Part model, mm, in its own coordinate system. Face numbers are marked on the shaded views. A direction names the side the tool comes from. Round coordinates to 2 decimals unless told otherwise and drop trailing zeros. Order: outer loops, then holes, each group sorted by start corner. A loop starts at its lowest first (then second) coordinate and runs counter-clockwise, first axis right, second up. Notation, with made-up numbers: (-25, 75) -> (33, 75) arc R9 cw to (33, 87) -> close; hole circle Ø7 at (-11, 72.25). An arc over 180 degrees is marked (long way). Use CSV: the item, a comma, the result in double quotes.
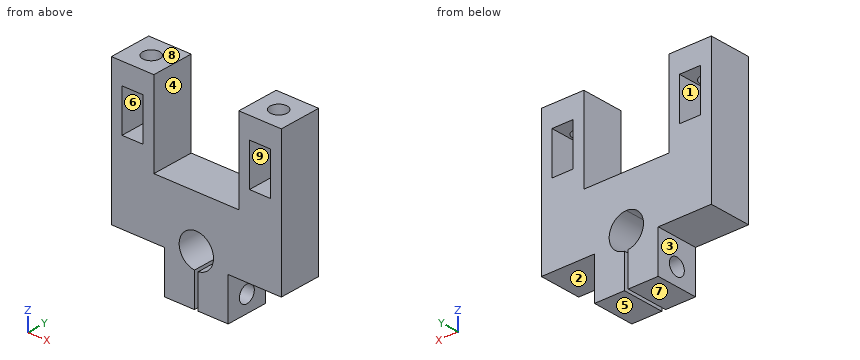
```python
from build123d import *

# Parameters (mm, degrees)
BOSS_EXTRUDE1_DEPTH = 10
SKETCH2_R           = 2
CUT_EXTRUDE1_DEPTH  = 15
SKETCH3_R           = 2
CUT_EXTRUDE2_DEPTH  = 11
SKETCH4_W           = 40
SKETCH4_H           = 24
BOSS_EXTRUDE2_DEPTH = 10
SKETCH5_R           = 4.04
CUT_EXTRUDE3_DEPTH  = 41.693979899
SKETCH6_W           = 0.9
SKETCH6_H           = 12
CUT_EXTRUDE4_DEPTH  = 41.693979899
SKETCH8_R           = 2
CUT_EXTRUDE5_DEPTH  = 40
SKETCH9_W           = 12.5
SKETCH9_H           = 10
CUT_EXTRUDE6_DEPTH  = 40
SKETCH10_W          = 5
SKETCH10_H          = 10
CUT_EXTRUDE7_DEPTH  = 10


with BuildPart() as part:
    # Sketch1 → Boss-Extrude1 (new body)
    with BuildSketch(Plane(origin=(0, 0, 0), x_dir=(1, 0, 0), z_dir=(0, 1, 0))):
        Polygon((-20, -10), (-20, 20), (20, 20), (20, -10), (10, -10), (10, 10), (-10, 10), (-10, -10), align=None)
    extrude(amount=BOSS_EXTRUDE1_DEPTH)

    # Sketch2 → Cut-Extrude1 (cut)
    with BuildSketch(Plane.XY.offset(10)):
        with Locations((-15, 5)):
            Circle(SKETCH2_R)
        with Locations((15, 5)):
            Circle(SKETCH2_R)
    extrude(amount=-CUT_EXTRUDE1_DEPTH, mode=Mode.SUBTRACT)

    # Sketch3 → Cut-Extrude2 (cut)
    with BuildSketch(Plane.XY.offset(-10)):
        with Locations((0, 5)):
            Circle(SKETCH3_R)
    extrude(amount=-CUT_EXTRUDE2_DEPTH, mode=Mode.SUBTRACT)

    # Sketch4 → Boss-Extrude2 (add, through all)
    with BuildSketch(Plane(origin=(0, 10, 0), x_dir=(1, 0, 0), z_dir=(0, 1, 0))):
        with Locations((0, 22)):
            Rectangle(SKETCH4_W, SKETCH4_H)
    extrude(amount=-BOSS_EXTRUDE2_DEPTH)

    # Sketch5 → Cut-Extrude3 (cut, through all)
    with BuildSketch(Plane(origin=(0, 10, 0), x_dir=(1, 0, 0), z_dir=(0, 1, 0))):
        with Locations(Location((0, 22, 0), (0, 0, 270))):
            Circle(SKETCH5_R)
    extrude(amount=-CUT_EXTRUDE3_DEPTH, mode=Mode.SUBTRACT)

    # Sketch6 → Cut-Extrude4 (cut, through all)
    with BuildSketch(Plane(origin=(0, 10, 0), x_dir=(1, 0, 0), z_dir=(0, 1, 0))):
        with Locations((0, 28)):
            Rectangle(SKETCH6_W, SKETCH6_H)
    extrude(amount=-CUT_EXTRUDE4_DEPTH, mode=Mode.SUBTRACT)

    # Sketch8 → Cut-Extrude5 (cut)
    with BuildSketch(Plane.ZY.offset(20)):
        with Locations((-30, 5)):
            Circle(SKETCH8_R)
    extrude(amount=-CUT_EXTRUDE5_DEPTH, mode=Mode.SUBTRACT)

    # Sketch9 → Cut-Extrude6 (cut)
    with BuildSketch(Plane(origin=(0, 10, 0), x_dir=(1, 0, 0), z_dir=(0, 1, 0))):
        with Locations((13.75, 29)):
            Rectangle(SKETCH9_W, SKETCH9_H)
        with Locations((-13.75, 29)):
            Rectangle(SKETCH9_W, SKETCH9_H)
    extrude(amount=-CUT_EXTRUDE6_DEPTH, mode=Mode.SUBTRACT)

    # Sketch10 → Cut-Extrude7 (cut)
    with BuildSketch(Plane(origin=(0, 10, 0), x_dir=(1, 0, 0), z_dir=(0, 1, 0))):
        with Locations((-15, 0)):
            Rectangle(SKETCH10_W, SKETCH10_H)
        with Locations((15, 0)):
            Rectangle(SKETCH10_W, SKETCH10_H)
    extrude(amount=-CUT_EXTRUDE7_DEPTH, mode=Mode.SUBTRACT)


solid = part.part
```
(1) Cut at B-B, the plane y = 7.75. Give the cut face in (x, z), then the cut area to 3 significant figures.
Reply:
outline,"(-20, -24) -> (-7.5, -24) -> (-7.5, -34) -> (-0.45, -34) -> (-0.45, -26.01) arc R4.04 cw (long way) to (0.45, -26.01) -> (0.45, -34) -> (7.5, -34) -> (7.5, -24) -> (20, -24) -> (20, 10) -> (10, 10) -> (10, -10) -> (-10, -10) -> (-10, 10) -> (-20, 10) -> close; hole (-17.5, -5) -> (-12.5, -5) -> (-12.5, 5) -> (-17.5, 5) -> close; hole (12.5, -5) -> (17.5, -5) -> (17.5, 5) -> (12.5, 5) -> close"
area,"952 mm2"
(2) Cut at A-A, the plane z = -9. Give the cut face in (x, y).
Reply:
outline,"(-20, 0) -> (-10, 0) -> (-10, 10) -> (-20, 10) -> close; (10, 0) -> (20, 0) -> (20, 10) -> (10, 10) -> close"
(3) Cut at D-D, the plane z = -30. Give the cut face in (x, y), then the cut area to 3 significant figures.
Reply:
outline,"(-7.5, 0) -> (-0.45, 0) -> (-0.45, 3) -> (-7.5, 3) -> close; (-7.5, 7) -> (-0.45, 7) -> (-0.45, 10) -> (-7.5, 10) -> close; (0.45, 0) -> (7.5, 0) -> (7.5, 3) -> (0.45, 3) -> close; (0.45, 7) -> (7.5, 7) -> (7.5, 10) -> (0.45, 10) -> close"
area,"84.6 mm2"
(4) Drop flat-ended pins along their axis: P1, Ø1, axis at x = -1.5, z = -14.5, coming from the -Y side; P2, Ø3, axis at x = -12.5, y = 4.5, coming from the -Z side. Give the stop position or say it passes through.
Reply:
P1,"y = 0"
P2,"z = -24"
(5) Cut at C-C, the plane x = 15. Give the cut face in (y, z).
Reply:
outline,"(0, -24) -> (10, -24) -> (10, -5) -> (0, -5) -> close; (0, 5) -> (3, 5) -> (3, 10) -> (0, 10) -> close; (7, 5) -> (10, 5) -> (10, 10) -> (7, 10) -> close"
(6) Which spindle directions (+Z, -Z, +X, -X, +Y, -Y) get a long thin tool onto all of the face, cutting with end or side? Do the marked faces 1, 2, 3, 4 and 5. Say none if no direction does.
Reply:
face 1,"+Y, -Y"
face 2,"-Z, +X, +Y, -Y"
face 3,"-Z, -X, +Y, -Y"
face 4,"+Z, +Y, -Y"
face 5,"-Z, +X, -X, +Y, -Y"
(7) Probe probe 1 along X at (y, z) = (3.75, 0.5); probe 2 along X at (y, z) = (9.25, 5.5); probe 3 along Z at (x, y) = (-15, 8). List the from-to ranges inside material, lowest first. Write a range as [from, to].
Reply:
probe 1,"[-20, -17.5], [-12.5, -10], [10, 12.5], [17.5, 20]"
probe 2,"[-20, -10], [10, 20]"
probe 3,"[-24, -5], [5, 10]"
(8) Pull direction Z, two halves, no side cores. Call the marked faces 6, 7, 8 and 9: released by +Z, released by -Z, zero draft, split by the parting line, or undercut.
Reply:
face 6,"undercut"
face 7,"released by -Z"
face 8,"released by +Z"
face 9,"undercut"
